Build history of the part. All positions in model axes, mm. Give positions to 0.01 mm unless a question says otherwise; leave off trailing zeros. Order: outer loops, then holes, each group sorted by start corner. A loop starts at its lowest first (then second) coordinate and runs counter-clockwise, first axis right, second up. Notation, with made-up numbers: (-37.5, 48.25) -> (-5.5, 48.25) arc R15 ccw to (-5.5, 56.25) -> close; hole circle Ø10 at (-13, 4). An arc over 180 degrees is marked (long way). Write item = value, one per line. Start each with the question number.
from build123d import *

# Parameters (mm, degrees)
SKETCH_W      = 130
SKETCH_H      = 50
PAD_DEPTH     = 2
SKETCH001_R   = 9.5
SKETCH001_R_2 = 7.75
SKETCH001_R_3 = 7.25
SKETCH001_R_4 = 5.5
PAD001_DEPTH  = 20


with BuildPart() as part:
    # Sketch → Pad (new body)
    with BuildSketch(Plane.XY):
        Rectangle(SKETCH_W, SKETCH_H)
    extrude(amount=PAD_DEPTH)

    # Sketch001 (on Face6 of Pad) → Pad001 (join)
    with BuildSketch(Plane.XY.offset(2)):
        with Locations((-50, 12.5)):
            Circle(SKETCH001_R)
        with Locations((-50, 12.5)):
            Circle(SKETCH001_R_2, mode=Mode.SUBTRACT)
        with Locations((-30, 12.5)):
            Circle(SKETCH001_R)
        with Locations((-30, 12.5)):
            Circle(SKETCH001_R_2, mode=Mode.SUBTRACT)
        with Locations((-10, 12.5)):
            Circle(SKETCH001_R)
        with Locations((-10, 12.5)):
            Circle(SKETCH001_R_2, mode=Mode.SUBTRACT)
        with Locations((10, 12.5)):
            Circle(SKETCH001_R)
        with Locations((10, 12.5)):
            Circle(SKETCH001_R_2, mode=Mode.SUBTRACT)
        with Locations((30, 12.5)):
            Circle(SKETCH001_R)
        with Locations((30, 12.5)):
            Circle(SKETCH001_R_2, mode=Mode.SUBTRACT)
        with Locations((50, 12.5)):
            Circle(SKETCH001_R)
        with Locations((50, 12.5)):
            Circle(SKETCH001_R_2, mode=Mode.SUBTRACT)
        with Locations((-50, -12.5)):
            Circle(SKETCH001_R_3)
        with Locations((-50, -12.5)):
            Circle(SKETCH001_R_4, mode=Mode.SUBTRACT)
        with Locations((-30, -12.5)):
            Circle(SKETCH001_R_3)
        with Locations((-30, -12.5)):
            Circle(SKETCH001_R_4, mode=Mode.SUBTRACT)
        with Locations((-10, -12.5)):
            Circle(SKETCH001_R_3)
        with Locations((-10, -12.5)):
            Circle(SKETCH001_R_4, mode=Mode.SUBTRACT)
        with Locations((10, -12.5)):
            Circle(SKETCH001_R_3)
        with Locations((10, -12.5)):
            Circle(SKETCH001_R_4, mode=Mode.SUBTRACT)
        with Locations((30, -12.5)):
            Circle(SKETCH001_R_3)
        with Locations((30, -12.5)):
            Circle(SKETCH001_R_4, mode=Mode.SUBTRACT)
        with Locations((50, -12.5)):
            Circle(SKETCH001_R_3)
        with Locations((50, -12.5)):
            Circle(SKETCH001_R_4, mode=Mode.SUBTRACT)
    extrude(amount=PAD001_DEPTH)


solid = part.part
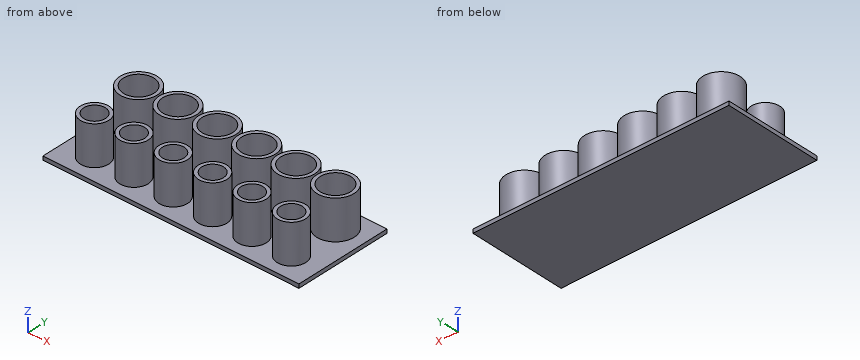
(1) Cut at A-A, the plane z = 15. Give the number of separate pieces and of enclosed holes in the cut face, plus the area to 3 significant figures.
(2) Wall check: line 1 (Y direction, x = 50, z = 11); line 2 (Y direction, x = 45, z = 10); line 3 (Z direction, x = 43.5, y = -1). Give the ranges that are in metal, low to high. Write a range as [from, to].
(3) Cut at B-B, the plane x = -30. Give the cut face in (y, z), plus the area to 3 significant figures.
(4) Flat gauge pins, fed straight in: P1, Ø4, axis at y = -14, z = 16.5, coming from the +X side; P2, Ø10, axis at x = 31, z = 9, coming from the +Y side; P3, Ø3.5, axis at x = 51.5, y = -11.5, coming from the +Z side. Where does each tip first touch, or does it go through?
(5) Cut at D-D, the plane x = 49. Give the cut face in (y, z).
(6) Cut at C-C, the plane y = -21. Give the cut face in (x, z), plus the area to 3 significant figures.
Results:
q1.separate_pieces = 12
q1.enclosed_holes = 12
q1.area = 990 mm2
q2.line_1 = [-19.75, -18], [-7, -5.25], [3, 4.75], [20.25, 22]
q2.line_2 = [-17.75, -14.79], [-10.21, -7.25], [4.42, 6.58], [18.42, 20.58]
q2.line_3 = [0, 2]
q3.outline = (-25, 0) -> (25, 0) -> (25, 2) -> (22, 2) -> (22, 22) -> (20.25, 22) -> (20.25, 2) -> (4.75, 2) -> (4.75, 22) -> (3, 22) -> (3, 2) -> (-5.25, 2) -> (-5.25, 22) -> (-7, 22) -> (-7, 2) -> (-18, 2) -> (-18, 22) -> (-19.75, 22) -> (-19.75, 2) -> (-25, 2) -> close
q3.area = 240 mm2
q4.P1 = 57.25
q4.P2 = 22
q4.P3 = 2
q5.outline = (-25, 0) -> (25, 0) -> (25, 2) -> (21.95, 2) -> (21.95, 22) -> (20.19, 22) -> (20.19, 2) -> (4.81, 2) -> (4.81, 22) -> (3.05, 22) -> (3.05, 2) -> (-5.32, 2) -> (-5.32, 22) -> (-7.09, 22) -> (-7.09, 2) -> (-17.91, 2) -> (-17.91, 22) -> (-19.68, 22) -> (-19.68, 2) -> (-25, 2) -> close
q6.outline = (-65, 0) -> (65, 0) -> (65, 2) -> (-65, 2) -> close
q6.area = 260 mm2
